Part model, mm, in its own coordinate system. A direction names the side the tool comes from. Round coordinates to 2 decimals unless told otherwise and drop trailing zeros. Loops run counter-clockwise (first coordinate to the right, second up) from the corner with the lowest first, then second, coordinate; pieces in that order, holes last.
1) Band-saw the part on B-B, the plane y = 10.5. Write the cut outline in (x, z).
2) Mould opens along Z. For faces 1 (the flat face through (0, 12.6, 0)), 2 (the cylindrical face through (1.73, 3.72, 7.81)), 3 (the cylindrical face through (6.863, 3.443, -1.376)) say: +Z half, -Z half, draft (parallel to the pull), parting line (faces both ways), or undercut.
3) Band-saw the part on A-A, the plane y = 2.75. State how many separate pieces and enclosed holes the cut face has, then the cut area to 3 significant figures.
4) 3-axis set-ups, long thin cutter, end or side, ignore diameter. For faces 4 (the flat face through (-4.9, 0.3, 5.3)), 5 (the cylindrical face through (2.17, 7.24, -1.52)): which of +Z, -Z, +X, -X, +Y, -Y reach the whole face in a straight line?
5) Probe line 1 (Z direction, x = 0, y = 4); line 2 (Z direction, x = 3, y = 7.25); line 3 (X direction, y = 3.5, z = 1). List the from-to ranges inside material, lowest first.
6) Drop flat-ended pins along their axis: P1, Ø7, axis at x = -2, z = -3.5, coming from the +Y side; P2, Ø1.6, axis at x = -3.5, y = 7.5, coming from the +Z side; P3, Ø4.5, axis at x = -3, z = -0.5, coming from the -Y side; P4, Ø2.5, axis at x = -6, z = 0, coming from the +Y side. Give the stop position or say it passes through.
Autodesk Inventor part; units mm, degrees
ref_plane "YZ Plane" through (0, 0, 0) normal (1, 0, 0) x (0, 1, 0)
ref_plane "XZ Plane" through (0, 0, 0) normal (0, 1, 0) x (-1, 0, 0)
ref_plane "XY Plane" through (0, 0, 0) normal (0, 0, 1) x (1, 0, 0)
sketch "Sketch1" plane through (0, 0, 0) normal (0, 1, 0) x (-1, 0, 0)
  circle A0 centre (0, 0) radius 8
  dimension "d0" = 16
extrude "Extrusion1" add sketch "Sketch1" along normal blind 8
sketch "Sketch2" plane through (0, 8, 0) normal (0, 1, 0) x (1, 0, 0)
  circle A0 centre (0, 0) radius 8
  circle A1 centre (0, 0) radius 2
  dimension "d3" = 4
extrude "Extrusion2" add sketch "Sketch2" along normal blind 4.6 contours A1
sketch "Sketch3" plane through (0, 0, 0) normal (0, -1, 0) x (1, 0, 0)
  circle A0 centre (0, 0) radius 8
  circle A1 centre (0, 0) radius 7.5
  dimension "d6" = 15
extrude "Extrusion3" cut sketch "Sketch3" against normal blind 6.5 contours A1
sketch "Sketch4" plane through (0, 6.5, 0) normal (0, -1, 0) x (1, 0, 0)
  circle A0 centre (0, 0) radius 7.5
  circle A1 centre (0, 0) radius 7
  line L0 (0, 0) -> (7.5, 0)
  circle A2 centre (0, 0) radius 7.5
  line L1 (0, 0) -> (6.9038, -2.9305)
  point P0 (6.4435, -2.7351)
  point P1 (6.9038, -2.9305)
  point P2 (7, 0)
  dimension "d9" = 14
  dimension "d10" = 23
extrude "Extrusion4" add sketch "Sketch4" along normal blind 6.2 contours A0 L1 A1 L0 picked at (6.8601, -2.5496)
pattern_circular "Circular Pattern1" count 10 over 360 about axis through (0, 0, 0) along (0, 1, 0) of "Extrusion4"
sketch "Sketch5" plane through (0, 8, 0) normal (0, 1, 0) x (1, 0, 0)
  circle A0 centre (0, 0) radius 2.5
  circle A1 centre (0, 0) radius 6.5
  line L0 (-10, -1) -> (-10, 1)
  line L1 (-10, 1) -> (10, 1)
  line L2 (10, 1) -> (10, -1)
  line L3 (10, -1) -> (-10, -1)
  line L4 (-10, -1) -> (10, 1) construction
  line L5 (-10, 1) -> (10, -1) construction
  line L6 (0, 0) -> (3.25, 5.6292)
  line L7 (0, 0) -> (-6.5, 0)
  line L8 (-5.866, -8.1603) -> (-4.134, -9.1603)
  line L9 (-4.134, -9.1603) -> (5.866, 8.1603)
  line L10 (5.866, 8.1603) -> (4.134, 9.1603)
  line L11 (4.134, 9.1603) -> (-5.866, -8.1603)
  line L12 (-5.866, -8.1603) -> (5.866, 8.1603) construction
  line L13 (-4.134, -9.1603) -> (4.134, 9.1603) construction
  point P0 (0.2796, 2.4843)
  point P1 (2.3453, 6.0621)
  point P2 (-6.4226, 1)
  point P3 (-2.2913, 1)
  dimension "d16" = 5
  dimension "d17" = 13
  dimension "d18" = 2
  dimension "d19" = 20
  dimension "d20" = 120
  dimension "d21" = 2
  dimension "d22" = 20
extrude "Extrusion5" cut sketch "Sketch5" against normal blind 6.2 contours A0 L1 A1 L11
pattern_circular "Circular Pattern2" count 3 over 360 about axis through (0, 8, 0) along (0, -1, 0) of "Extrusion5"
fillet "Fillet1" radius 1.5 2 edges at (-6.4226, 7.25, -1) (2.3453, 7.25, -6.0621)
pattern_circular "Circular Pattern3" count 3 over 360 about axis through (0, 8, 0) along (0, 1, 0) of "Fillet1"
fillet "Fillet2" radius 1 2 edges at (-2.2913, 7.25, -1) (0.2796, 7.25, -2.4843)
pattern_circular "Circular Pattern4" count 3 over 360 about axis through (0, 8, 0) along (0, 1, 0) of "Fillet2"
chamfer "Chamfer1" distance 0.8 angle 30 1 edges at (8, 8, 0) measured on face at (-6.1962, 8, 0)
sketch "Sketch6" plane through (0, 6.5, 0) normal (0, -1, 0) x (1, 0, 0)
  arc A0 (0, 6.5) -> (-5.6292, 3.25) centre (0, 0) ccw
  arc A1 (1.299, 4.25) -> (0, 6.5) centre (0, 5) ccw
  line L0 (1.299, 4.25) -> (0.5701, 2.9875)
  arc A2 (-0.2114, 2.491) -> (0.5701, 2.9875) centre (-0.2959, 3.4875) ccw
  arc A3 (-0.2114, 2.491) -> (-2.0516, 1.4286) centre (0, 0) ccw
  arc A4 (-2.8723, 1) -> (-2.0516, 1.4286) centre (-2.8723, 2) ccw
  line L1 (-2.8723, 1) -> (-4.3301, 1)
  arc A5 (-5.6292, 3.25) -> (-4.3301, 1) centre (-4.3301, 2.5) ccw
  arc A6 (5.6292, -3.25) -> (5.6292, 3.25) centre (0, 0) ccw
  arc A7 (3.0311, -3.25) -> (5.6292, -3.25) centre (4.3301, -2.5) ccw
  line L2 (3.0311, -3.25) -> (2.3022, -1.9875)
  arc A8 (2.263, -1.0625) -> (2.3022, -1.9875) centre (3.1682, -1.4875) ccw
  arc A9 (2.263, -1.0625) -> (2.263, 1.0625) centre (0, 0) ccw
  arc A10 (2.3022, 1.9875) -> (2.263, 1.0625) centre (3.1682, 1.4875) ccw
  line L3 (2.3022, 1.9875) -> (3.0311, 3.25)
  arc A11 (5.6292, 3.25) -> (3.0311, 3.25) centre (4.3301, 2.5) ccw
  arc A12 (-5.6292, -3.25) -> (0, -6.5) centre (0, 0) ccw
  arc A13 (-4.3301, -1) -> (-5.6292, -3.25) centre (-4.3301, -2.5) ccw
  line L4 (-4.3301, -1) -> (-2.8723, -1)
  arc A14 (-2.0516, -1.4286) -> (-2.8723, -1) centre (-2.8723, -2) ccw
  arc A15 (-2.0516, -1.4286) -> (-0.2114, -2.491) centre (0, 0) ccw
  arc A16 (0.5701, -2.9875) -> (-0.2114, -2.491) centre (-0.2959, -3.4875) ccw
  line L5 (0.5701, -2.9875) -> (1.299, -4.25)
  arc A17 (0, -6.5) -> (1.299, -4.25) centre (0, -5) ccw
  line L6 (7.3078, 1.6871) -> (6.8206, 1.5747)
  arc A18 (6.8206, 1.5747) -> (5.6631, 4.1145) centre (0, 0) ccw
  line L7 (5.6631, 4.1145) -> (6.0676, 4.4084)
  arc A19 (6.0676, 4.4084) -> (4.9204, 5.6603) centre (0, 0) ccw
  line L8 (4.9204, 5.6603) -> (4.5924, 5.283)
  arc A20 (4.5924, 5.283) -> (2.1631, 6.6574) centre (0, 0) ccw
  line L9 (2.1631, 6.6574) -> (2.3176, 7.1329)
  arc A21 (2.3176, 7.1329) -> (0.6537, 7.4715) centre (0, 0) ccw
  line L10 (0.6537, 7.4715) -> (0.6101, 6.9734)
  arc A22 (0.6101, 6.9734) -> (-2.1631, 6.6574) centre (0, 0) ccw
  line L11 (-2.1631, 6.6574) -> (-2.3176, 7.1329)
  arc A23 (-2.3176, 7.1329) -> (-3.8628, 6.4288) centre (0, 0) ccw
  line L12 (-3.8628, 6.4288) -> (-3.6053, 6.0002)
  arc A24 (-3.6053, 6.0002) -> (-5.6631, 4.1145) centre (0, 0) ccw
  line L13 (-5.6631, 4.1145) -> (-6.0676, 4.4084)
  arc A25 (-6.0676, 4.4084) -> (-6.9038, 2.9305) centre (0, 0) ccw
  line L14 (-6.9038, 2.9305) -> (-6.4435, 2.7351)
  arc A26 (-6.4435, 2.7351) -> (-7, 0) centre (0, 0) ccw
  line L15 (-7, 0) -> (-7.5, 0)
  arc A27 (-7.5, 0) -> (-7.3078, -1.6871) centre (0, 0) ccw
  line L16 (-7.3078, -1.6871) -> (-6.8206, -1.5747)
  arc A28 (-6.8206, -1.5747) -> (-5.6631, -4.1145) centre (0, 0) ccw
  line L17 (-5.6631, -4.1145) -> (-6.0676, -4.4084)
  arc A29 (-6.0676, -4.4084) -> (-4.9204, -5.6603) centre (0, 0) ccw
  line L18 (-4.9204, -5.6603) -> (-4.5924, -5.283)
  arc A30 (-4.5924, -5.283) -> (-2.1631, -6.6574) centre (0, 0) ccw
  line L19 (-2.1631, -6.6574) -> (-2.3176, -7.1329)
  arc A31 (-2.3176, -7.1329) -> (-0.6537, -7.4715) centre (0, 0) ccw
  line L20 (-0.6537, -7.4715) -> (-0.6101, -6.9734)
  arc A32 (-0.6101, -6.9734) -> (2.1631, -6.6574) centre (0, 0) ccw
  line L21 (2.1631, -6.6574) -> (2.3176, -7.1329)
  arc A33 (2.3176, -7.1329) -> (3.8628, -6.4288) centre (0, 0) ccw
  line L22 (3.8628, -6.4288) -> (3.6053, -6.0002)
  arc A34 (3.6053, -6.0002) -> (5.6631, -4.1145) centre (0, 0) ccw
  line L23 (5.6631, -4.1145) -> (6.0676, -4.4084)
  arc A35 (6.0676, -4.4084) -> (6.9038, -2.9305) centre (0, 0) ccw
  line L24 (6.9038, -2.9305) -> (6.4435, -2.7351)
  arc A36 (6.4435, -2.7351) -> (7, 0) centre (0, 0) ccw
  line L25 (7, 0) -> (7.5, 0)
  arc A37 (7.5, 0) -> (7.3078, 1.6871) centre (0, 0) ccw
  circle A38 centre (0, 0) radius 1.5
  dimension "d39" = 3
extrude "Extrusion6" add sketch "Sketch6" along normal blind 5 contours A38
sketch "Sketch7" plane through (0, 8, 0) normal (0, 1, 0) x (1, 0, 0)
  circle A0 centre (0, 0) radius 2
  arc A1 (0, 6.5) -> (-5.6292, 3.25) centre (0, 0) ccw
  arc A2 (1.299, 4.25) -> (0, 6.5) centre (0, 5) ccw
  line L0 (1.299, 4.25) -> (0.5701, 2.9875)
  arc A3 (-0.2114, 2.491) -> (0.5701, 2.9875) centre (-0.2959, 3.4875) ccw
  arc A4 (-0.2114, 2.491) -> (-2.0516, 1.4286) centre (0, 0) ccw
  arc A5 (-2.8723, 1) -> (-2.0516, 1.4286) centre (-2.8723, 2) ccw
  line L1 (-2.8723, 1) -> (-4.3301, 1)
  arc A6 (-5.6292, 3.25) -> (-4.3301, 1) centre (-4.3301, 2.5) ccw
  arc A7 (5.6292, -3.25) -> (5.6292, 3.25) centre (0, 0) ccw
  arc A8 (3.0311, -3.25) -> (5.6292, -3.25) centre (4.3301, -2.5) ccw
  line L2 (3.0311, -3.25) -> (2.3022, -1.9875)
  arc A9 (2.263, -1.0625) -> (2.3022, -1.9875) centre (3.1682, -1.4875) ccw
  arc A10 (2.263, -1.0625) -> (2.263, 1.0625) centre (0, 0) ccw
  arc A11 (2.3022, 1.9875) -> (2.263, 1.0625) centre (3.1682, 1.4875) ccw
  line L3 (2.3022, 1.9875) -> (3.0311, 3.25)
  arc A12 (5.6292, 3.25) -> (3.0311, 3.25) centre (4.3301, 2.5) ccw
  arc A13 (-5.6292, -3.25) -> (0, -6.5) centre (0, 0) ccw
  arc A14 (-4.3301, -1) -> (-5.6292, -3.25) centre (-4.3301, -2.5) ccw
  line L4 (-4.3301, -1) -> (-2.8723, -1)
  arc A15 (-2.0516, -1.4286) -> (-2.8723, -1) centre (-2.8723, -2) ccw
  arc A16 (-2.0516, -1.4286) -> (-0.2114, -2.491) centre (0, 0) ccw
  arc A17 (0.5701, -2.9875) -> (-0.2114, -2.491) centre (-0.2959, -3.4875) ccw
  line L5 (0.5701, -2.9875) -> (1.299, -4.25)
  arc A18 (0, -6.5) -> (1.299, -4.25) centre (0, -5) ccw
  circle A19 centre (0, 0) radius 7.2
  line L6 (0, 0) -> (-6, 0)
  circle A20 centre (-6, 0) radius 0.75
  dimension "d42" = 6
  dimension "d43" = 1.5
extrude "Extrusion7" cut sketch "Sketch7" against normal blind 5 contours A20
pattern_circular "Circular Pattern5" count 3 over 360 about axis through (0, 8, 0) along (0, 1, 0) of "Extrusion7"
properties part number "motor_1608_outer"
Reported:
1. outline: circle Ø4 at (0, 0)
2. face 1: draft
2. face 2: parting line
2. face 3: undercut
3. separate pieces: 2
3. enclosed holes: 1
3. area: 46.0 mm2
4. face 4: -Y
4. face 5: +Y, -Y
5. line 1: z = -8 to -7, -1.5 to 1.5, 7 to 8
5. line 2: z = -7.42 to -5.95, -4.45 to -3.2, 3.2 to 4.45, 5.95 to 7.42
5. line 3: x = -7.94 to -6.93, -1.12 to 1.12, 7.43 to 7.94
6. P1: stops at y = 12.6
6. P2: stops at z = 7.53
6. P3: stops at y = 1.5
6. P4: stops at y = 8
